Part model, mm, in its own coordinate system. A direction names the side the tool comes from. Round coordinates to 2 decimals unless told otherwise and drop trailing zeros. Write each loop counter-clockwise with the first axis right and the second up, starting at its lowest first coordinate (ties: lowest second). Pieces come first, ordered by that corner, then holes. Notation, with made-up numbers: M 56,37.25 L 110,37.25 A26 ccw 110,60.25 Z; hole C -3,45 d8. An arc over 180 degrees is marked long. Use one line per item in the form item = value. Start each with the question number.
Item 1: Cut at C-C, the plane z = 20. Give the cut face in (x, y).
Item 2: Which spindle directions (+Z, -Z, +X, -X, +Y, -Y) get a long thin tool onto all of the face, cutting with end or side? Do faces 4 (the face through (12, 21, 29.5)), 5 (the face through (4.119, 18.548, 13.592)). Say none if no direction does.
Item 3: Mould opens along X. For faces 1 (the face through (-12, 21, 27)), 2 (the face through (-6, 17, 2.5)), 3 (the face through (2.799, -21.317, 13.661)) say: +X half, -X half, draft (parallel to the pull), parting line (faces both ways), or undercut.
Item 4: Probe L1, parallel to Y at x = 0, z = 10.25; L2, parallel to Z at x = -24, y = 8; L3, parallel to Y at x = -6, z = 25.75. List the from-to ranges inside material, lowest first.
Item 5: Cut at A-A, the plane y = 0. Give the cut face in (x, z), then the cut area to 3 significant figures.
Item 6: Flat gauge pins, fed straight in: pin 1 Ø2 at (y, z) = (8.5, 12) entering from -X; pin 2 Ø1 at (y, z) = (-8, 7.5) entering from +X; pin 3 Ø8 at (x, z) = (-17.5, 16) entering from -Y. Where does each tip first touch, or does it go through?
from build123d import *


with BuildPart() as part:
    # Sketch1 → Revolve1 (revolve)
    with BuildSketch(Plane(origin=(0, 0, 0), x_dir=(0, 0, -1), z_dir=(1, 0, 0)), mode=Mode.PRIVATE) as revolve1_sk:
        with BuildLine():
            Line((0, 17.4625), (0, 19.5))
            ThreePointArc((0, 19.5), (-0.585786438, 20.914213562), (-2, 21.5))
            Line((-2, 21.5), (-25, 21.5))
            ThreePointArc((-25, 21.5), (-26.414213562, 22.085786438), (-27, 23.5))
            Line((-27, 23.5), (-27, 31.5))
            Line((-27, 31.5), (-29.5, 31.5))
            Line((-29.5, 31.5), (-29.5, 23.5))
            ThreePointArc((-29.5, 23.5), (-28.181980515, 20.318019485), (-25, 19))
            Line((-25, 19), (-2.5, 19))
            Line((-2.5, 19), (-2.5, 17.4625))
            Line((-2.5, 17.4625), (0, 17.4625))
        make_face()
    revolve(revolve1_sk.sketch.rotate(Axis((0, 0, 0), (0, 0, 1)), 90), axis=Axis((0, 0, 0), (0, 0, 1)))


solid = part.part
Model answer:
q1.outline = C 0,0 d43; hole C 0,0 d38
q2.face_4 = +Z, +X, -X, +Y, -Y
q2.face_5 = +Z
q3.face_1 = draft
q3.face_2 = undercut
q3.face_3 = parting line
q4.L1 = -21.5 to -19, 19 to 21.5
q4.L2 = 27 to 29.5
q4.L3 = -20.8 to -18.09, 18.09 to 20.8
q5.outline = M -31.5,27 L -23.5,27 A2 cw -21.5,25 L -21.5,2 A2 ccw -19.5,0 L -17.46,0 L -17.46,2.5 L -19,2.5 L -19,25 A4.5 ccw -23.5,29.5 L -31.5,29.5 Z; M 17.46,0 L 19.5,0 A2 ccw 21.5,2 L 21.5,25 A2 cw 23.5,27 L 31.5,27 L 31.5,29.5 L 23.5,29.5 A4.5 ccw 19,25 L 19,2.5 L 17.46,2.5 Z
q5.area = 196 mm²
q6.pin_1 = -20.15
q6.pin_2 = 20.15
q6.pin_3 = -16.73
